The model under review builds one solid part; all positions refer to its coordinate system, in mm. Face numbers are marked on the shaded views. A direction names the side the tool comes from. Round coordinates to 2 decimals unless told otherwise and drop trailing zeros. Order: outer loops, then holes, each group sorted by start corner. A loop starts at its lowest first (then second) coordinate and runs counter-clockwise, first axis right, second up. Notation, with made-up numbers: M -11,-26 L 19,-26 A26 ccw 19,8 Z; hole C 89,9.5 d4. An arc over 180 degrees is marked long. Answer as CSV lines item,"result". Start each with the question number.
from build123d import *

# Parameters (mm, degrees)
SKETCH1_W           = 22.8
SKETCH1_H           = 16
BOSS_EXTRUDE1_DEPTH = 12
SKETCH2_W           = 32.5
SKETCH2_H           = 12
MOUNTING_DEPTH      = 2.4
SKETCH4_W           = 22.8
SKETCH4_H           = 12
BOSS_EXTRUDE4_DEPTH = 4
SKETCH6_R           = 2.7
SKETCH6_R_2         = 6
BOSS_EXTRUDE5_DEPTH = 4.2
SKETCH7_R           = 2.4
BOSS_EXTRUDE6_DEPTH = 2.8
SKETCH8_R           = 1
CUT_EXTRUDE1_DEPTH  = 2.8
SKETCH9_W           = 10
SKETCH9_H           = 13
CUT_EXTRUDE2_DEPTH  = 1


with BuildPart() as part:
    # Sketch1 → Boss-Extrude1 (new body)
    with BuildSketch(Plane.XY):
        Rectangle(SKETCH1_W, SKETCH1_H)
    extrude(amount=BOSS_EXTRUDE1_DEPTH)

    # Sketch2 → mounting (add)
    with BuildSketch(Plane(origin=(0, 8, 0), x_dir=(1, 0, 0), z_dir=(0, 1, 0))):
        with Locations((0, -6)):
            Rectangle(SKETCH2_W, SKETCH2_H)
    extrude(amount=MOUNTING_DEPTH)

    # Sketch4 → Boss-Extrude4 (add)
    with BuildSketch(Plane(origin=(0, 10.4, 0), x_dir=(1, 0, 0), z_dir=(0, 1, 0))):
        with Locations((0, -6)):
            Rectangle(SKETCH4_W, SKETCH4_H)
    extrude(amount=BOSS_EXTRUDE4_DEPTH)

    # Sketch6 → Boss-Extrude5 (add)
    with BuildSketch(Plane(origin=(0, 14.4, 0), x_dir=(1, 0, 0), z_dir=(0, 1, 0))):
        with Locations((-0.9, -6)):
            Circle(SKETCH6_R)
        with Locations((5.4, -6)):
            Circle(SKETCH6_R_2)
        with BuildLine():
            Line((0.04182867, -3.3), (-0.9, -3.3))
            ThreePointArc((-0.9, -3.3), (-0.458336611, -3.336368372), (-0.028571429, -3.44449374))
            ThreePointArc((-0.028571429, -3.44449374), (0.006144751, -3.37201112), (0.04182867, -3.3))
        make_face()
    extrude(amount=BOSS_EXTRUDE5_DEPTH)

    # Sketch7 → Boss-Extrude6 (add)
    with BuildSketch(Plane(origin=(0, 18.6, 0), x_dir=(1, 0, 0), z_dir=(0, 1, 0))):
        with Locations((5.4, -6)):
            Circle(SKETCH7_R)
    extrude(amount=BOSS_EXTRUDE6_DEPTH)

    # Sketch8 → Cut-Extrude1 (cut)
    with BuildSketch(Plane(origin=(0, 10.4, 0), x_dir=(1, 0, 0), z_dir=(0, 1, 0))):
        with Locations((-14.25, -6)):
            Circle(SKETCH8_R)
        with BuildLine():
            ThreePointArc((-14.25, -7), (-15.25, -6), (-14.25, -5))
            Line((-14.25, -5), (-16.25, -5))
            Line((-16.25, -5), (-16.25, -7))
            Line((-16.25, -7), (-14.25, -7))
        make_face()
        with BuildLine():
            ThreePointArc((15.25, -6), (14.957106781, -6.707106781), (14.25, -7))
            Line((14.25, -7), (16.25, -7))
            Line((16.25, -7), (16.25, -5))
            Line((16.25, -5), (14.25, -5))
            ThreePointArc((14.25, -5), (14.957106781, -5.292893219), (15.25, -6))
        make_face()
        with Locations((14.25, -6)):
            Circle(SKETCH8_R)
    extrude(amount=-CUT_EXTRUDE1_DEPTH, mode=Mode.SUBTRACT)

    # Sketch9 → Cut-Extrude2 (cut)
    with BuildSketch(Plane(origin=(0, 0, 0), x_dir=(-1, 0, 0), z_dir=(0, 0, -1))):
        Rectangle(SKETCH9_W, SKETCH9_H)
    extrude(amount=-CUT_EXTRUDE2_DEPTH, mode=Mode.SUBTRACT)


solid = part.part
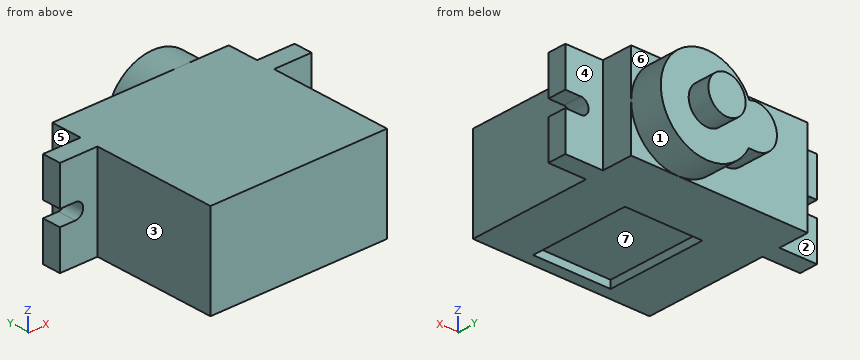
Item 1: For pin 1 (0.6 mm diameter, centred on x = 15.5, y = 9, fed in from -Z); pin 2 (6 mm diameter, centred on y = 14.5, z = 10, fed in from +X); pin 3 (4 mm diameter, centred on x = 14.5, z = 6.5, fed in from +Y); pin 4 (2.5 mm diameter, centred on x = -13, z = 5.5, fed in from -Y), all flat-tipped, find the tip position at first contact; note any pin that passes through.
Item 2: The part is to be moulded in two halves that separate along Y. For the marked faces 5, 6 and 7, say which applies: +Y half, -Y half, draft (parallel to the pull), parting line (faces both ways), or undercut.
Item 3: Consider section C-C (x = -0.5). State the section outline as (y, z) points.
Item 4: Consider section B-B (y = -5). State the section outline as (x, z) points.
Item 5: Wall thickness on probe 1 along Y at (x, z) = (-7, 5.75); probe 2 along Y at (x, z) = (6, 11); probe 3 along X at (y, z) = (-4, 1.25): over which ranges is each line inside the solid? List them lowest first. Write a range as [from, to].
Item 6: Tool access review of the marked faces 1, 2, 3 and 4: name each direction out of +Z, -Z, +X, -X, +Y, -Y from which nothing blocks a thin tool from reaching the whole face with its end or side.
Item 7: Consider section D-D (z = 10.75). State the section outline as (x, y) points.
Reported:
1,pin 1,"stops at z = 0"
1,pin 2,"stops at x = 11.4"
1,pin 3,"stops at y = 10.4"
1,pin 4,"stops at y = 8"
2,face 5,"draft"
2,face 6,"+Y half"
2,face 7,"undercut"
3,outline,"M -8,0 L -6.5,0 L -6.5,1 L 6.5,1 L 6.5,0 L 14.4,0 L 14.4,3.3 L 18.6,3.3 L 18.6,8.67 L 14.4,8.67 L 14.4,12 L -8,12 Z"
4,outline,"M -11.4,0 L -5,0 L -5,1 L 5,1 L 5,0 L 11.4,0 L 11.4,12 L -11.4,12 Z"
5,probe 1,"y = [-8, 14.4]"
5,probe 2,"y = [-8, 18.6]"
5,probe 3,"x = [-11.4, 11.4]"
6,face 1,"+Y"
6,face 2,"+Z, -Z, -X, +Y"
6,face 3,"+Z, -Z, -X, -Y"
6,face 4,"+Z, -Z, +X, +Y"
7,outline,"M -16.25,8 L -11.4,8 L -11.4,-8 L 11.4,-8 L 11.4,8 L 16.25,8 L 16.25,10.4 L 11.4,10.4 L 11.4,14.4 L 9.07,14.4 L 9.07,18.6 L 1.73,18.6 L 1.73,14.4 L -11.4,14.4 L -11.4,10.4 L -16.25,10.4 Z"
